from build123d import *

# Parameters (mm, degrees)
SKETCH1_R           = 10
SKETCH1_R_2         = 7.5
BOSS_EXTRUDE1_DEPTH = 20
SKETCH2_R           = 7.5
BOSS_EXTRUDE2_DEPTH = 6


with BuildPart() as part:
    # Sketch1 → Boss-Extrude1 (new body)
    with BuildSketch(Plane.XY):
        with Locations((-123, -48)):
            Circle(SKETCH1_R)
        with Locations((-123, -48)):
            Circle(SKETCH1_R_2, mode=Mode.SUBTRACT)
    extrude(amount=BOSS_EXTRUDE1_DEPTH)

    # Sketch2 → Boss-Extrude2 (add)
    with BuildSketch(Plane(origin=(0, 0, 0), x_dir=(-1, 0, 0), z_dir=(0, 0, -1))):
        with BuildLine():
            Line((111, -28), (135, -28))
            ThreePointArc((135, -28), (140.656854249, -30.343145751), (143, -36))
            Line((143, -36), (143, -60))
            ThreePointArc((143, -60), (140.656854249, -65.656854249), (135, -68))
            Line((135, -68), (111, -68))
            ThreePointArc((111, -68), (105.343145751, -65.656854249), (103, -60))
            Line((103, -60), (103, -36))
            ThreePointArc((103, -36), (105.343145751, -30.343145751), (111, -28))
        make_face()
        with Locations(Location((123, -48, 0), (0, 0, 180))):
            Circle(SKETCH2_R, mode=Mode.SUBTRACT)
    extrude(amount=-BOSS_EXTRUDE2_DEPTH)


solid = part.part
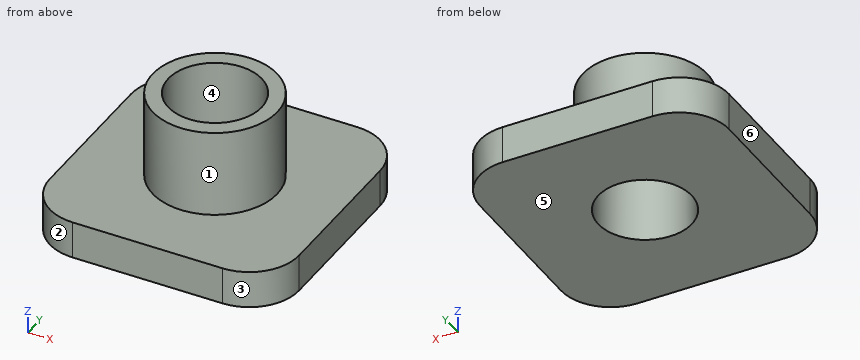
Can you work these out from the model? Positions are in its coordinate system, mm. Face numbers are marked on the shaded views. A direction names the side the tool comes from. Give positions to 0.01 mm unless a question says otherwise; leave off trailing zeros. Write each loop counter-clockwise with the first axis right and the second up, starting at its lowest first coordinate (ties: lowest second). Pieces come first, ordered by that corner, then holes. Notation, with made-up numbers: M -30,-6.5 L -18,-6.5 A30 cw -18,32.5 Z; hole C 21,45 d9. An arc over 180 degrees is marked long. Answer in a Markdown table with one row per item. Add a question column.
Item 1: Imagine slicing it at B-B, the plane y = -48. Write out the boundary of the cut face in (x, z).
Item 2: We'd pull the mould along X, two halves only. Please class the marked faces 3, 4, 5 and 6: released by +X, released by -X, zero draft, split by the parting line, or undercut.
Item 3: Please list where these lines run through material, in increasing order: L1, parallel to Y at x = -123, z = 11.25; L2, parallel to Y at x = -123, z = 5; L3, parallel to Z at x = -129.5, y = -64.
Item 4: On a 3-axis mill with a long thin cutter (end or side, diameter ignored), from which of +Z, -Z, +X, -X, +Y, -Y can I reach the whole of each face in a straight line? I mean the marked faces 1 and 2. Say none if no direction works.
Item 5: For pin 1 Ø1 at (x, y) = (-134.5, -45.5) entering from +Z; pin 2 Ø5 at (x, z) = (-111.5, 10) entering from +Y; pin 3 Ø4 at (y, z) = (-48.5, 9.5) entering from -X, each with a flat end and sliding along its axis, tell me the tip position at first contact or that it passes through.
Item 6: Imagine slicing it at C-C, the plane z = 2.75. Write out the boundary of the cut face in (x, y), plus the area to 3 significant figures.
Item 7: Imagine slicing it at A-A, the plane x = -123. Write out the boundary of the cut face in (y, z).
Item 8: Imagine slicing it at D-D, the plane z = 9.5. Write out the boundary of the cut face in (x, y).
Evaluation:
| question | item | result |
|---|---|---|
| 1 | outline | M -143,0 L -130.5,0 L -130.5,20 L -133,20 L -133,6 L -143,6 Z; M -115.5,0 L -103,0 L -103,6 L -113,6 L -113,20 L -115.5,20 Z |
| 2 | face 3 | released by +X |
| 2 | face 4 | undercut |
| 2 | face 5 | zero draft |
| 2 | face 6 | released by -X |
| 3 | L1 | y = -58 to -55.5, -40.5 to -38 |
| 3 | L2 | y = -68 to -55.5, -40.5 to -28 |
| 3 | L3 | z = 0 to 6 |
| 4 | face 1 | +Z |
| 4 | face 2 | +Z, -Z, -X, -Y |
| 5 | pin 1 | stops at z = 6 |
| 5 | pin 2 | stops at y = -43.64 |
| 5 | pin 3 | stops at x = -133 |
| 6 | outline | M -143,-60 A8 ccw -135,-68 L -111,-68 A8 ccw -103,-60 L -103,-36 A8 ccw -111,-28 L -135,-28 A8 ccw -143,-36 Z; hole C -123,-48 d15 |
| 6 | area | 1,370 mm² |
| 7 | outline | M -68,0 L -55.5,0 L -55.5,20 L -58,20 L -58,6 L -68,6 Z; M -40.5,0 L -28,0 L -28,6 L -38,6 L -38,20 L -40.5,20 Z |
| 8 | outline | C -123,-48 d20; hole C -123,-48 d15 |
